Geometry: see drawing. Coordinates: mm, zero at the bounding-box minimum. A direction names the side the tool comes from. Give positions to 0.01 mm unless a question says otherwise; leave off trailing zeros. Write each loop counter-clockwise with the first axis right and the second up, starting at its lowest first coordinate (ties: lowest second). Pieces come first, ordered by that corner, then holes. Notation, with made-up numbers: (36, -25) - (49, -25) arc R26 cw to (49, 5) - close; hole circle Ø6 at (-37, 44.5). An arc over 180 degrees is marked (long way). Use CSV: the item, a comma, the result in double quotes. Start each with the question number.
(1) Section A-A on y = 75.5. Output: boundary loops of the cut face in (x, z), and give its area (3 significant figures).
(2) Reachability of the marked faces 1, 2 and 3 from +Z, -Z, +X, -X, +Y, -Y: full face, straight path, thin tool, end or side. Return the list, or none.
(3) Line query: probe 1 along Z at (x, y) = (40.75, 75); probe 2 along X at (y, z) = (66.5, 7.25); probe 3 along Z at (x, y) = (39, 75). Output: solid intervals per line, ascending. Write a range as [from, to].
(4) First-contact query: pin 1 Ø1 at (x, z) = (10.5, 3.5) entering from -Y; pin 2 Ø2 at (x, z) = (20.5, 5) entering from -Y; pin 3 Ø6 at (y, z) = (71.5, 10) entering from -X. Flat tips, straight axial feed; report the tip coordinate or a pass-through.
(5) Section B-B on x = 20. Output: boundary loops of the cut face in (y, z).
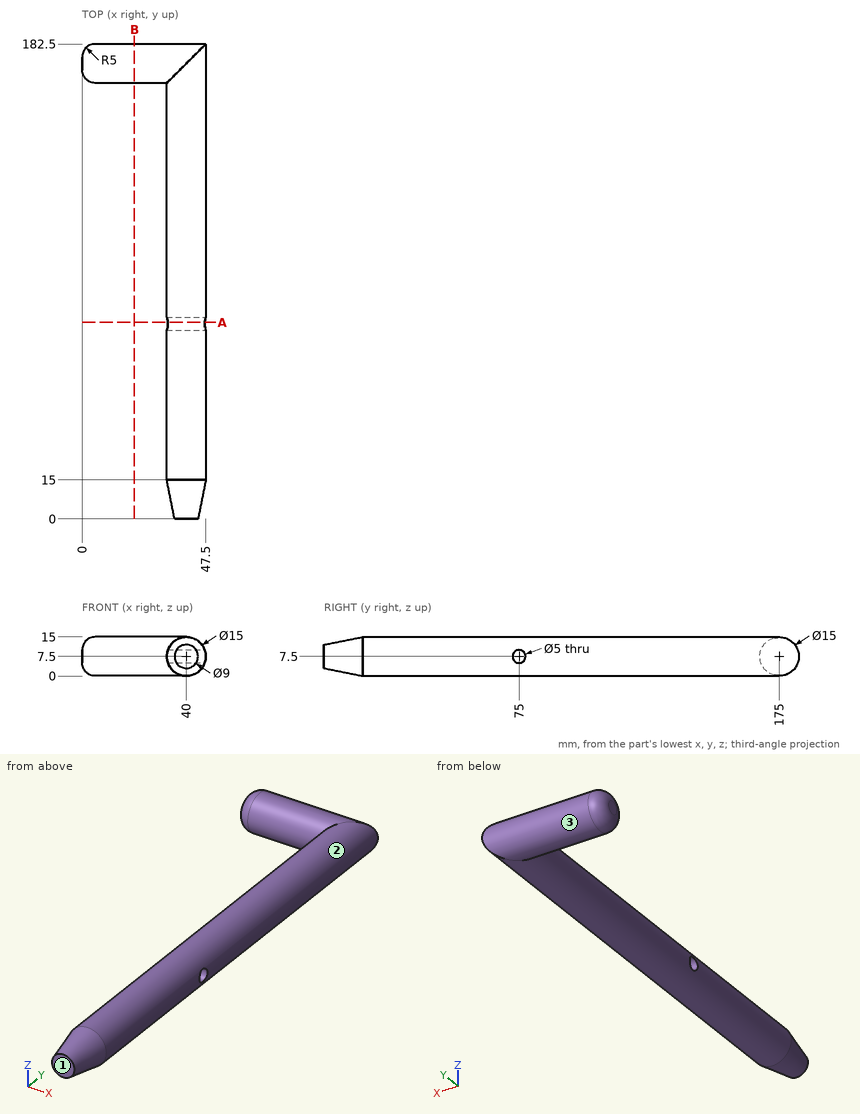
Check values:
1,outline,"(32.91, 5.05) arc R7.5 ccw to (47.09, 5.05) - close; (32.91, 9.95) - (47.09, 9.95) arc R7.5 ccw to start"
1,area,"105 mm²"
2,face 1,"+Z, -Z, +X, -X, -Y"
2,face 2,"-Y"
2,face 3,"-X"
3,probe 1,"z = [0.04, 5], [10, 14.96]"
3,probe 2,"x = [32.5, 47.5]"
3,probe 3,"z = [0.07, 5], [10, 14.93]"
4,pin 1,"stops at y = 168.37"
4,pin 2,"stops at y = 167.65"
4,pin 3,"stops at x = 32.5"
5,outline,"circle Ø15 at (175, 7.5)"
